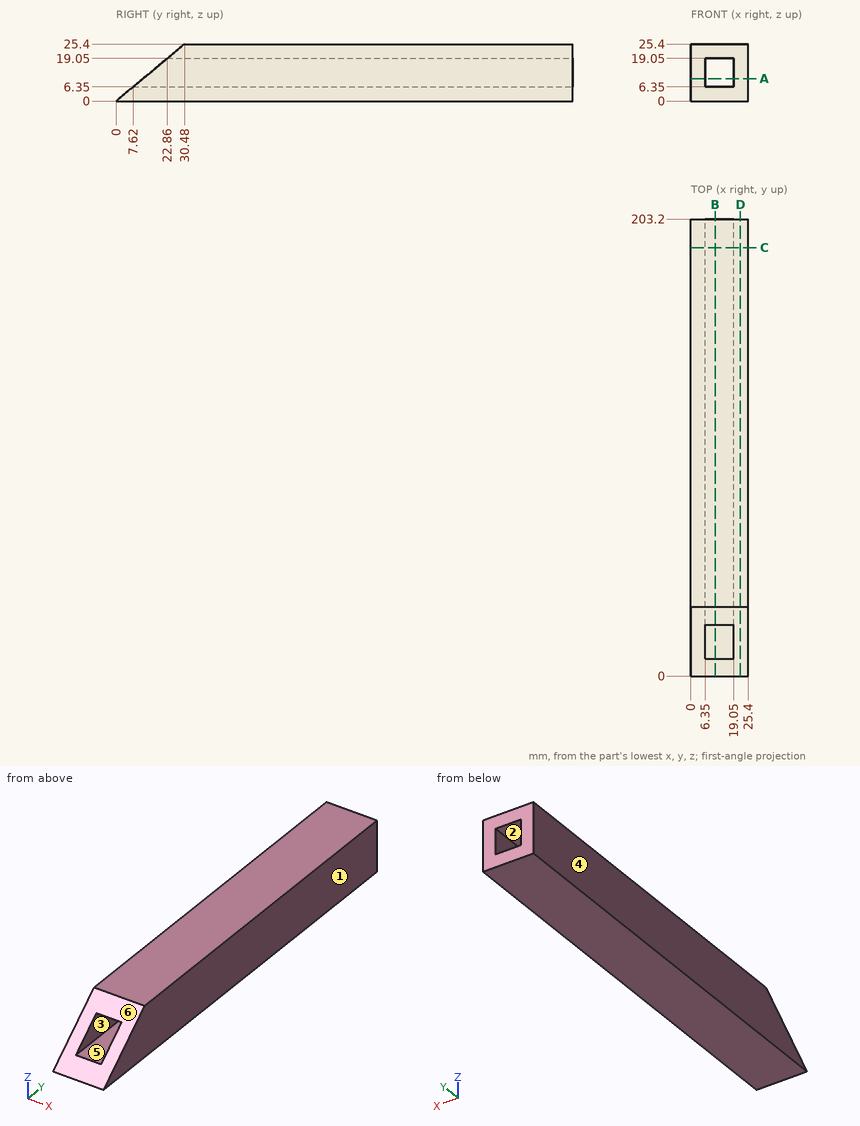
Here's the drawing with two shaded views (mm, measured from the low corner). I have some questions. A direction names the side the tool comes from. Give positions to 0.01 mm unless a question says otherwise; leave off trailing zeros. Write each loop counter-clockwise with the first axis right and the second up, starting at its lowest first coordinate (ties: lowest second). Pieces come first, ordered by that corner, then holes. Notation, with made-up numbers: (36, 6.25) - (80, 6.25) arc R28 ccw to (80, 28.25) - close; hole circle Ø4 at (9, 51.25). An arc over 180 degrees is marked (long way). Write item = value, one per line. Start each with the question number.
1. Imagine slicing it at D-D (x = 22). Please give me the cut outline in (y, z), and give its area (3 significant figures).
2. Please list where these lines run through material, in increasing order: line 1 (Z direction, x = 18.5, y = 119); line 2 (Y direction, x = 6, z = 23.5).
3. Imagine slicing it at B-B (x = 10.75). Please give me the cut outline in (y, z).
4. Imagine slicing it at C-C (y = 190.5). Please give me the cut outline in (x, z).
5. Imagine slicing it at A-A (z = 10). Please give me the cut outline in (x, y).
6. For pin 1 (3 mm diameter, centred on x = 12.5, z = 18.5, fed in from -Y), with a flat end and sliding along its axis, tell me the tip position at first contact or that it passes through.
7. On a 3-axis mill with a long thin cutter (end or side, diameter ignored), from which of +Z, -Z, +X, -X, +Y, -Y can I reach the whole of each face in a straight line? I mean the marked faces 1 and 2. Say none if no direction works.
8. Thinking about a two-plate mould opening in Z: for the marked faces 3, 4, 5 and 6, which applies, released by +Z, released by -Z, zero draft, split by the parting line, or undercut?
Worked answers:
q1.outline = (0, 0) - (203.2, 0) - (203.2, 25.4) - (30.48, 25.4) - close
q1.area = 4,770 mm2
q2.line_1 = 0 to 6.35, 19.05 to 25.4
q2.line_2 = 28.2 to 203.2
q3.outline = (0, 0) - (203.2, 0) - (203.2, 6.35) - (7.62, 6.35) - close; (22.86, 19.05) - (203.2, 19.05) - (203.2, 25.4) - (30.48, 25.4) - close
q4.outline = (0, 0) - (25.4, 0) - (25.4, 25.4) - (0, 25.4) - close; hole (6.35, 6.35) - (19.05, 6.35) - (19.05, 19.05) - (6.35, 19.05) - close
q5.outline = (0, 12) - (6.35, 12) - (6.35, 203.2) - (0, 203.2) - close; (19.05, 12) - (25.4, 12) - (25.4, 203.2) - (19.05, 203.2) - close
q6.pin_1 = 22.86
q7.face_1 = +Z, -Z, +X, +Y, -Y
q7.face_2 = +Y, -Y
q8.face_3 = undercut
q8.face_4 = zero draft
q8.face_5 = undercut
q8.face_6 = released by +Z
